Read the model definition and answer for the solid it produces. Units are mm, in the model's axes. A direction names the side the tool comes from. Round coordinates to 2 decimals unless told otherwise and drop trailing zeros. Loops run counter-clockwise (first coordinate to the right, second up) from the corner with the lowest first, then second, coordinate; pieces in that order, holes last. Notation, with made-up numbers: (9, 44.5) - (49, 44.5) arc R18 cw to (49, 79.5) - close; hole circle Ø1 at (30, 47.25). An arc over 180 degrees is marked (long way). Use CSV: the item, a comma, the result in double quotes. Start each with the question number.
1. Given pin 1 Ø5 at (x, y) = (11.14, 187) entering from -Z, flat-ended and moving along its own axis, determine where the tip first touches the part or whether it passes through.
2. Find section A-A (y = 31). Give the vertices of the cut face in (x, z).
3. Determine the mould class of faces 1 (the flat face through (0, 101, 2)), 2 (the flat face through (51, 0, 2)), 3 (the flat face through (72, 32.1, 2)) for opening direction X: +X half, -X half, draft (parallel to the pull), parting line (faces both ways), or undercut.
4. Find section C-C (x = 29). Give the vertices of the cut face in (y, z).
5. Consider line 1 along Y through (x, z) = (9.5, 1.4); line 2 along Y through (x, z) = (18, 0.9); line 3 along X through (y, z) = (203, 2.5). Determine where each line is inside the solid, lowest interval first.
6. A tool of negligible diameter and unlimited length cuts with its end or side. For faces 4 (the flat face through (20, 81, 2)), 5 (the cylindrical face through (48.2, 212.89, 2.03)), from which of +Z, -Z, +X, -X, +Y, -Y can it reach the whole face along a straight path? Write none if from no direction.
7. Find section B-B (x = 47). Give the vertices of the cut face in (y, z).
8. Find section D-D (y = 195). Give the vertices of the cut face in (x, z), and give its area (3 significant figures).
from build123d import *

# Parameters (mm, degrees)
ESBO_O1_R                = 12.5
ESBO_O1_R_2              = 1.5
ESBO_O1_R_3              = 2.5
RESSALTO_EXTRUS_O2_DEPTH = 4
FILETE1_R                = 10
ESBO_O2_R                = 1.5
ESBO_O2_R_2              = 2.6
ESBO_O2_R_3              = 3.05
CORTE_EXTRUS_O1_DEPTH    = 5
ESBO_O3_R                = 3
CORTE_EXTRUS_O2_DEPTH    = 5


with BuildPart() as part:
    # Esboço1 → Ressalto-extrusão2 (new body)
    with BuildSketch(Plane.XY):
        Polygon((0, 0), (0, 215), (50, 215), (100, 0), align=None)
        with Locations((25, 195)):
            Circle(ESBO_O1_R, mode=Mode.SUBTRACT)
        with Locations((25, 211)):
            Circle(ESBO_O1_R_2, mode=Mode.SUBTRACT)
        with Locations((38.856406461, 203)):
            Circle(ESBO_O1_R_2, mode=Mode.SUBTRACT)
        with Locations((38.856406461, 187)):
            Circle(ESBO_O1_R_2, mode=Mode.SUBTRACT)
        with Locations((25, 179)):
            Circle(ESBO_O1_R_2, mode=Mode.SUBTRACT)
        with Locations((11.143593539, 187)):
            Circle(ESBO_O1_R_2, mode=Mode.SUBTRACT)
        with Locations((11.143593539, 203)):
            Circle(ESBO_O1_R_2, mode=Mode.SUBTRACT)
        with Locations((18, 47)):
            Circle(ESBO_O1_R_3, mode=Mode.SUBTRACT)
        with BuildLine():
            Line((20, 95), (20, 66))
            ThreePointArc((20, 66), (20.878679656, 63.878679656), (23, 63))
            Line((23, 63), (61.03739436, 63))
            ThreePointArc((61.03739436, 63), (63.386715693, 64.134339454), (63.959418441, 66.679540484))
            Line((63.959418441, 66.679540484), (57.215232395, 95.679540484))
            ThreePointArc((57.215232395, 95.679540484), (56.15886886, 97.349321333), (54.293208314, 98))
            Line((54.293208314, 98), (23, 98))
            ThreePointArc((23, 98), (20.878679656, 97.121320344), (20, 95))
        make_face(mode=Mode.SUBTRACT)
        with BuildLine():
            Line((20, 40), (20, 23))
            ThreePointArc((20, 23), (20.878679656, 20.878679656), (23, 20))
            Line((23, 20), (71.03739436, 20))
            ThreePointArc((71.03739436, 20), (73.386715693, 21.134339454), (73.959418441, 23.679540484))
            Line((73.959418441, 23.679540484), (70.005930069, 40.679540484))
            ThreePointArc((70.005930069, 40.679540484), (68.949566534, 42.349321333), (67.083905988, 43))
            Line((67.083905988, 43), (23, 43))
            ThreePointArc((23, 43), (20.878679656, 42.121320344), (20, 40))
        make_face(mode=Mode.SUBTRACT)
    extrude(amount=RESSALTO_EXTRUS_O2_DEPTH)

    # Filete1
    filete1_edges = [part.edges().sort_by_distance(p)[0] for p in [
        (0, 215, 2),
        (50, 215, 2),
    ]]
    fillet(filete1_edges, radius=FILETE1_R)

    # Esboço2 → Corte-extrusão1 (cut, through all)
    with BuildSketch(Plane.XY.offset(4)):
        with Locations((9.5, 137)):
            Circle(ESBO_O2_R)
        with Locations((90.5, 14.5)):
            Circle(ESBO_O2_R_2)
        with Locations((9.5, 112)):
            Circle(ESBO_O2_R)
        with Locations((9.5, 152)):
            Circle(ESBO_O2_R_3)
        with Locations((59, 112)):
            Circle(ESBO_O2_R)
        with Locations((9.5, 14.5)):
            Circle(ESBO_O2_R_2)
        with BuildLine():
            Line((13.5, 161.71), (13.5, 166.71))
            ThreePointArc((13.5, 166.71), (15, 168.21), (16.5, 166.71))
            Line((16.5, 166.71), (16.5, 161.71))
            ThreePointArc((16.5, 161.71), (15, 160.21), (13.5, 161.71))
        make_face()
        with BuildLine():
            Line((33.5, 161.71), (33.5, 166.71))
            ThreePointArc((33.5, 166.71), (35, 168.21), (36.5, 166.71))
            Line((36.5, 166.71), (36.5, 161.71))
            ThreePointArc((36.5, 161.71), (35, 160.21), (33.5, 161.71))
        make_face()
    extrude(amount=-CORTE_EXTRUS_O1_DEPTH, mode=Mode.SUBTRACT)

    # Esboço3 → Corte-extrusão2 (cut, through all)
    with BuildSketch(Plane.XY.offset(4)):
        with Locations((70.759810426, 80.398555206)):
            Circle(ESBO_O3_R)
    extrude(amount=-CORTE_EXTRUS_O2_DEPTH, mode=Mode.SUBTRACT)


solid = part.part
Filled sheet:
1,pin 1,"stops at z = 0"
2,outline,"(0, 0) - (20, 0) - (20, 4) - (0, 4) - close; (72.26, 0) - (92.79, 0) - (92.79, 4) - (72.26, 4) - close"
3,face 1,"-X half"
3,face 2,"draft"
3,face 3,"undercut"
4,outline,"(0, 0) - (20, 0) - (20, 4) - (0, 4) - close; (43, 0) - (63, 0) - (63, 4) - (43, 4) - close; (98, 0) - (183.16, 0) - (183.16, 4) - (98, 4) - close; (206.84, 0) - (215, 0) - (215, 4) - (206.84, 4) - close"
5,line 1,"y = 0 to 11.9, 17.1 to 110.5, 113.5 to 135.5, 138.5 to 148.95, 155.05 to 214.99"
5,line 2,"y = 0 to 44.5, 49.5 to 184.64, 205.36 to 215"
5,line 3,"x = 0 to 9.64, 12.64 to 15.4, 34.6 to 37.36, 40.36 to 52.79"
6,face 4,"+Z, -Z"
6,face 5,"+Z, -Z, +X, +Y"
7,outline,"(0, 0) - (20, 0) - (20, 4) - (0, 4) - close; (43, 0) - (63, 0) - (63, 4) - (43, 4) - close; (98, 0) - (213.69, 0) - (213.69, 4) - (98, 4) - close"
8,outline,"(0, 0) - (12.5, 0) - (12.5, 4) - (0, 4) - close; (37.5, 0) - (54.65, 0) - (54.65, 4) - (37.5, 4) - close"
8,area,"119 mm²"
